Model file for the job. Use its own axes, mm. A direction names the side the tool comes from. Give positions to 0.01 mm unless a question says otherwise; leave off trailing zeros. Loops run counter-clockwise (first coordinate to the right, second up) from the corner with the lowest first, then second, coordinate; pieces in that order, holes last. Notation, with made-up numbers: M -20.5,36 L 24.5,36 A20 ccw 24.5,70 Z; hole C -31,15 d4. An arc over 180 degrees is marked long. Answer in a Markdown table with one row per item.
```python
from build123d import *

# Parameters (mm, degrees)
SKETCH1_R           = 30.1625
SKETCH1_R_2         = 23.8125
ID_2_DEPTH          = 25.4
SKETCH2_R           = 36.576
SKETCH2_R_2         = 30.1625
OD_DEPTH            = 50.8
SKETCH4_R           = 23.8125
BOSS_EXTRUDE3_DEPTH = 12.7


with BuildPart() as part:
    # Sketch1 → ID 2 (new body)
    with BuildSketch(Plane(origin=(0, 0, 0), x_dir=(1, 0, 0), z_dir=(0, 1, 0))):
        with Locations(Location((0, 0, 0), (0, 0, 270))):
            Circle(SKETCH1_R)
        with Locations(Location((0, 0, 0), (0, 0, 270))):
            Circle(SKETCH1_R_2, mode=Mode.SUBTRACT)
    extrude(amount=ID_2_DEPTH)

    # Sketch2 → OD (add)
    with BuildSketch(Plane.XZ):
        with Locations(Location((0, 0, 0), (0, 0, 270))):
            Circle(SKETCH2_R)
        with Locations(Location((0, 0, 0), (0, 0, 270))):
            Circle(SKETCH2_R_2, mode=Mode.SUBTRACT)
    extrude(amount=-OD_DEPTH)

    # Sketch4 → Boss-Extrude3 (add)
    with BuildSketch(Plane.XZ):
        Polygon((0, 98.552), (-98.552, 98.552), (-98.552, 0), (-98.552, -98.552), (0, -98.552), (98.552, -98.552), (98.552, 0), (98.552, 98.552), align=None)
        with Locations(Location((0, 0, 0), (0, 0, 90))):
            Circle(SKETCH4_R, mode=Mode.SUBTRACT)
    extrude(amount=-BOSS_EXTRUDE3_DEPTH)


solid = part.part
```
Q1. Drop flat-ended pins along their axis: pin 1 (1 mm diameter, centred on x = -49, z = 5, fed in from +Y); pin 2 (8 mm diameter, centred on x = 31.5, y = 19, fed in from +Z); pin 3 (10 mm diameter, centred on y = 37.5, z = -30.5, fed in from +X); pin 4 (6 mm diameter, centred on y = 14.5, z = 50, fed in from -X). Give the stop position or say it passes through.
Reported:
| item | result |
|---|---|
| pin 1 | y = 12.7 |
| pin 2 | z = 24.12 |
| pin 3 | x = 26.22 |
| pin 4 | x = -98.55 |
Q2. Mould opens along Z. For faces 3 (the face through (-1, 6, -98.552)), 4 (the face through (-32.45, 31.48, -16.88)), 5 (the face through (-98.552, 6, 1)), 6 (the face through (9.1, 25.4, 22.2)) say: released by +Z, released by -Z, zero draft, split by the parting line, or undercut.
Reported:
| item | result |
|---|---|
| face 3 | released by -Z |
| face 4 | split by the parting line |
| face 5 | zero draft |
| face 6 | undercut |
Q3. Saw through at B-B (z = 0). Give the cut face in (x, y), and give its area (3 significant figures).
Reported:
| item | result |
|---|---|
| outline | M -98.55,0 L -23.81,0 L -23.81,25.4 L -30.16,25.4 L -30.16,50.8 L -36.58,50.8 L -36.58,12.7 L -98.55,12.7 Z; M 23.81,0 L 98.55,0 L 98.55,12.7 L 36.58,12.7 L 36.58,50.8 L 30.16,50.8 L 30.16,25.4 L 23.81,25.4 Z |
| area | 2,550 mm² |
Q4. 3-axis set-ups, long thin cutter, end or side, ignore diameter. For faces 1 (the face through (1.326, 37.922, 30.133)), 2 (the face through (1, 6, 98.552)): which of +Z, -Z, +X, -X, +Y, -Y reach the whole face in a straight line?
Reported:
| item | result |
|---|---|
| face 1 | +Y |
| face 2 | +Z, +X, -X, +Y, -Y |
Q5. Probe probe 1 along X at (y, z) = (37, 0); probe 2 along X at (y, z) = (11, 0); probe 3 along Y at (x, z) = (57, 24). List the from-to ranges inside material, lowest first.
Reported:
| item | result |
|---|---|
| probe 1 | -36.58 to -30.16, 30.16 to 36.58 |
| probe 2 | -98.55 to -23.81, 23.81 to 98.55 |
| probe 3 | 0 to 12.7 |
Q6. Saw through at D-D (x = 68). Give the cut face in (y, z).
Reported:
| item | result |
|---|---|
| outline | M 0,-98.55 L 12.7,-98.55 L 12.7,98.55 L 0,98.55 Z |
Q7. Saw through at C-C (y = 42.5). Give the cut face in (x, z) (1 decimal).
Reported:
| item | result |
|---|---|
| outline | C 0,0 d73.2; hole C 0,0 d60.3 |
Q8. Saw through at A-A (x = 0). Give the cut face in (y, z).
Reported:
| item | result |
|---|---|
| outline | M 0,-98.55 L 12.7,-98.55 L 12.7,-36.58 L 50.8,-36.58 L 50.8,-30.16 L 25.4,-30.16 L 25.4,-23.81 L 0,-23.81 Z; M 0,23.81 L 25.4,23.81 L 25.4,30.16 L 50.8,30.16 L 50.8,36.58 L 12.7,36.58 L 12.7,98.55 L 0,98.55 Z |
